For this review, take the finished solid that the model builds, in its own axes (mm). A direction names the side the tool comes from. Give positions to 0.01 mm unless a question says otherwise; leave off trailing zeros. Order: outer loops, then holes, each group sorted by start corner. A loop starts at its lowest first (then second) coordinate and runs counter-clockwise, first axis right, second up.
Item 1: For probe 1 along Z at (x, y) = (0, 3.25) (3 decimals); probe 2 along X at (y, z) = (5.75, -8.25); probe 3 along Z at (x, y) = (6.25, 2), list the stretches that pass through material, from the lowest coordinate up.
Item 2: Consider section D-D (z = 7.75). Give the boundary of the cut face in (x, y), plus the area to 3 significant figures.
Item 3: Consider section B-B (z = 0). Give the boundary of the cut face in (x, y) (3 decimals), plus the area to 3 significant figures.
Item 4: Consider section A-A (x = 0). Give the boundary of the cut face in (y, z) (3 decimals).
Item 5: For P1, Ø1.5, axis at x = -5, y = 2, coming from the +Z side; P2, Ø1, axis at x = 3, y = 4, coming from the +Z side; P3, Ø10, axis at x = 7, z = -1, coming from the -Y side; P4, Ø2, axis at y = 5.5, z = 5.5, coming from the +X side, all flat-tipped, find the tip position at first contact; note any pin that passes through.
Item 6: Machinability: for faces 1 (the flat face through (-6.46, 3.22, -9.02)), 2 (the flat face through (0, 3, 12.7)), 3 (the flat face through (1.796, 3.219, 10.991)), 4 (the flat face through (10.94, 3.22, 1.81)), 5 (the flat face through (-10.94, 3.22, -1.81)), which of the approach directions +Z, -Z, +X, -X, +Y, -Y give a long, thin tool a straight path to every point of the face, cutting with its end or side? Answer none if there is none.
Item 7: The part is to be moulded in two halves that separate along Z. For faces 6 (the cylindrical face through (0.69, 3.13, 3.1)), 7 (the flat face through (8.97, 3.22, -8.99)), 8 (the flat face through (-3, 6.35, -3)), say which applies: released by +Z, released by -Z, zero draft, split by the parting line, or undercut.
Autodesk Inventor part; units mm, degrees
ref_plane "YZ Plane" through (0, 0, 0) normal (1, 0, 0) x (0, 1, 0)
ref_plane "XZ Plane" through (0, 0, 0) normal (0, 1, 0) x (-1, 0, 0)
ref_plane "XY Plane" through (0, 0, 0) normal (0, 0, 1) x (1, 0, 0)
sketch "Sketch1" plane through (0, 0, 0) normal (0, 1, 0) x (-1, 0, 0)
  circle A0 centre (0, 0) radius 9.525
  circle A1 centre (0, 0) radius 3.175
  dimension "d0" = 19.05
  dimension "d1" = 6.35
extrude "Extrusion1" add sketch "Sketch1" along normal blind 6.35
sketch "Sketch2" plane through (0, 6.35, 0) normal (0, 1, 0) x (1, 0, 0)
  circle A0 centre (0, 0) radius 9.525
  line L0 (0, -9.525) -> (0, -12.7)
  line L1 (0, -12.7) -> (-1.27, -12.7)
  line L2 (0, -12.7) -> (1.27, -12.7)
  line L3 (-2.3368, -9.2339) -> (2.3368, -9.2339)
  line L4 (1.27, -12.7) -> (2.3368, -9.2339)
  line L5 (-2.3368, -9.2339) -> (-1.27, -12.7)
  dimension "d4" = 3.175
  dimension "d5" = 1.27
  dimension "d6" = 1.27
  dimension "d12" = 4.6736
extrude "Extrusion2" add sketch "Sketch2" against normal blind 6.35 contours A0 L0 L1 L5 | L4 L2 L0 A0
pattern_circular "Circular Pattern1" count 8 over 360 about axis through (0, 0, 0) along (0, 1, 0) of "Extrusion2"
properties part number "drivenGear"
Resolved:
1. probe 1: z = -12.7 to -3.175, 3.175 to 12.7
1. probe 2: x = -9.71 to -5.01, -4.76 to 4.76, 5.01 to 9.71
1. probe 3: z = -8.91 to 8.91
2. outline: (-9.7, 0) - (9.7, 0) - (9.7, 6.35) - (-9.7, 6.35) - close
2. area: 123 mm2
3. outline: (-12.7, 0) - (-3.175, 0) - (-3.175, 6.35) - (-12.7, 6.35) - close; (3.175, 0) - (12.7, 0) - (12.7, 6.35) - (3.175, 6.35) - close
3. area: 121 mm2
4. outline: (0, -12.7) - (6.35, -12.7) - (6.35, -3.175) - (0, -3.175) - close; (0, 3.175) - (6.35, 3.175) - (6.35, 12.7) - (0, 12.7) - close
5. P1: stops at z = 8.64
5. P2: stops at z = 9.19
5. P3: stops at y = 0
5. P4: stops at x = 9.04
6. face 1: -Z, +Y, -Y
6. face 2: +Z, +X, -X, +Y, -Y
6. face 3: +Z, +Y, -Y
6. face 4: +X, +Y, -Y
6. face 5: -X, +Y, -Y
7. face 6: undercut
7. face 7: released by -Z
7. face 8: zero draft
